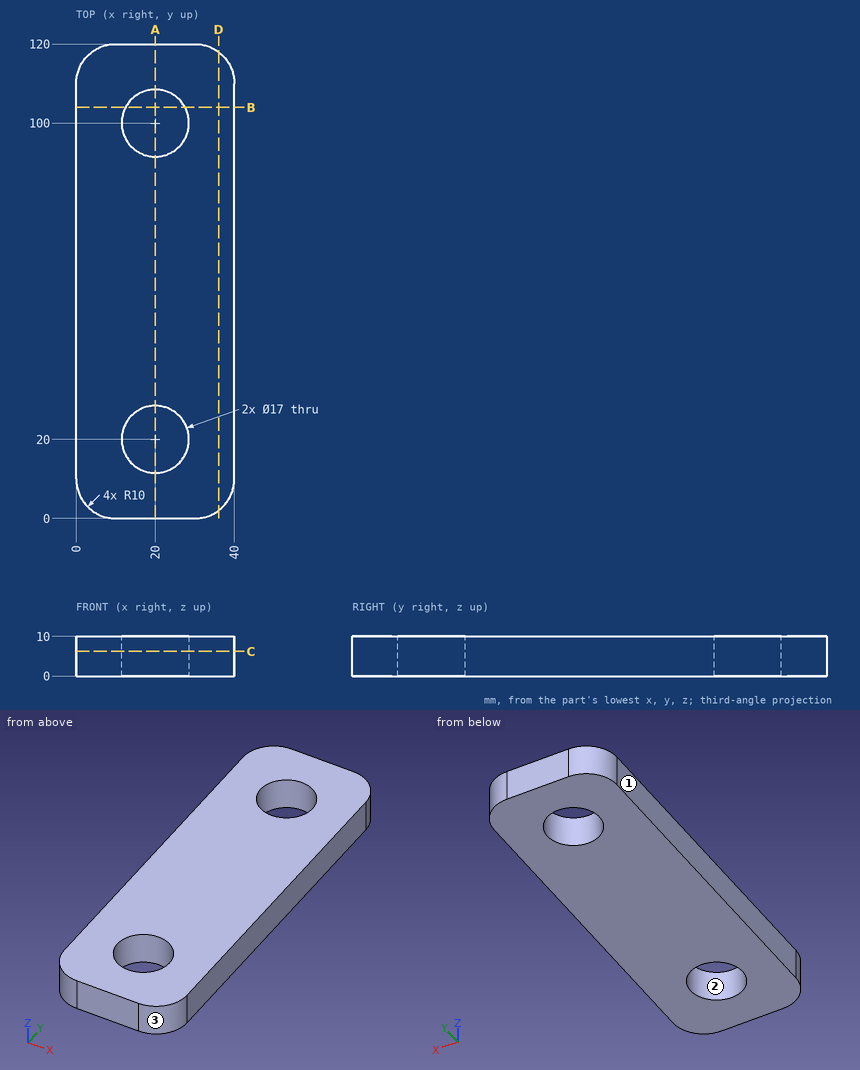
The drawing under review shows one solid part. Ordinate dimensions are in mm from its lowest x, y, z. Give positions to 0.01 mm unless a question says otherwise; leave off trailing zeros. Write each loop counter-clockwise with the first axis right and the second up, starting at its lowest first coordinate (ties: lowest second). Pieces come first, ordered by that corner, then holes. Notation, with made-up numbers: M 41.25,2.5 L 95.25,2.5 A22 ccw 95.25,19.5 Z; hole C -0.5,36 d4. An arc over 180 degrees is marked long. Write each question's results on one line, items separated by ' | '. Start each with the question number.
1. For probe 1 along Y at (x, z) = (20, 7.25); probe 2 along X at (y, z) = (20.5, 6.25); probe 3 along X at (y, z) = (21, 8), list the stretches that pass through material, from the lowest coordinate up. Write a range as [from, to].
2. We need section B-B (y = 104). Write out the cut boundary in (x, z), and give its area (3 significant figures).
3. We need section A-A (x = 20). Write out the cut boundary in (y, z).
4. We need section D-D (x = 36). Write out the cut boundary in (y, z), and give its area (3 significant figures).
5. Insertion check: pin 1 Ø3 at (x, z) = (7.5, 1.5) entering from +Y; pin 2 Ø2 at (x, z) = (31.5, 2.5) entering from -Y. Each pin has a flat end and moves straight along its axis. Give the tip position at first contact, or say it passes through.
6. Mouldability with a two-part tool opening along X and no side actions: class the marked faces 1, 2 and 3 as released by +X, released by -X, zero draft, split by the parting line, or undercut.
7. We need section C-C (z = 6.25). Write out the cut boundary in (x, y).
Results found:
1) probe 1: y = [0, 11.5], [28.5, 91.5], [108.5, 120] | probe 2: x = [0, 11.51], [28.49, 40] | probe 3: x = [0, 11.56], [28.44, 40]
2) outline: M 0,0 L 12.5,0 L 12.5,10 L 0,10 Z; M 27.5,0 L 40,0 L 40,10 L 27.5,10 Z | area: 250 mm^2
3) outline: M 0,0 L 11.5,0 L 11.5,10 L 0,10 Z; M 28.5,0 L 91.5,0 L 91.5,10 L 28.5,10 Z; M 108.5,0 L 120,0 L 120,10 L 108.5,10 Z
4) outline: M 2,0 L 118,0 L 118,10 L 2,10 Z | area: 1,160 mm^2
5) pin 1: stops at y = 119.95 | pin 2: stops at y = 0.01
6) face 1: released by -X | face 2: undercut | face 3: released by +X
7) outline: M 0,10 A10 ccw 10,0 L 30,0 A10 ccw 40,10 L 40,110 A10 ccw 30,120 L 10,120 A10 ccw 0,110 Z; hole C 20,20 d17; hole C 20,100 d17
